```python
from build123d import *

# Parameters (mm, degrees)
SKETCH1_W                      = 16
SKETCH1_H                      = 40
BOSS_EXTRUDE1_DEPTH            = 30
F_3_8_0_3750_DOWEL_HOLE1_D     = 9.525
F_1_8_0_1250_DOWEL_HOLE1_D     = 3.175
SKETCH7_W                      = 10
SKETCH7_H                      = 40
CUT_EXTRUDE1_DEPTH             = 15
F_3_16_0_1875_DIAMETER_HOLE1_D = 4.7625
SKETCH10_W                     = 16
SKETCH10_H                     = 23.65
CUT_EXTRUDE2_DEPTH             = 15
FILLET1_R                      = 10


with BuildPart() as part:
    # Sketch1 → Boss-Extrude1 (new body)
    with BuildSketch(Plane.XY):
        with Locations((0, -10)):
            Rectangle(SKETCH1_W, SKETCH1_H)
    extrude(amount=BOSS_EXTRUDE1_DEPTH)

    # 3/8 (0.3750) Dowel Hole1 (through all)
    with Locations(Plane.XY.offset(30)):
        with Locations((0, 0)):
            Hole(F_3_8_0_3750_DOWEL_HOLE1_D / 2)

    # 1/8 (0.1250) Dowel Hole1 (through all)
    with Locations(Plane.ZY.offset(8)):
        with Locations((7.5, 0)):
            Hole(F_1_8_0_1250_DOWEL_HOLE1_D / 2)

    # Sketch7 → Cut-Extrude1 (cut)
    with BuildSketch(Plane.XY.offset(30)):
        with Locations((0, -10)):
            Rectangle(SKETCH7_W, SKETCH7_H)
    extrude(amount=-CUT_EXTRUDE1_DEPTH, mode=Mode.SUBTRACT)

    # 3/16 (0.1875) Diameter Hole1 (through all)
    with Locations(Plane.ZY.offset(8)):
        with Locations((22, -2), (22, -23.7)):
            Hole(F_3_16_0_1875_DIAMETER_HOLE1_D / 2)

    # Sketch10 → Cut-Extrude2 (cut)
    with BuildSketch(Plane(origin=(0, 0, 0), x_dir=(-1, 0, 0), z_dir=(0, 0, -1))):
        with Locations((0, -18.175)):
            Rectangle(SKETCH10_W, SKETCH10_H)
    extrude(amount=-CUT_EXTRUDE2_DEPTH, mode=Mode.SUBTRACT)

    # Fillet1
    fillet1_edges = [part.edges().sort_by_distance(p)[0] for p in [
        (6.5, 10, 30),
        (6.5, -30, 30),
        (-6.5, 10, 30),
        (-6.5, -30, 30),
    ]]
    fillet(fillet1_edges, radius=FILLET1_R)


solid = part.part
```
Build history of the part. All positions in model axes, mm. A direction names the side the tool comes from. Coordinates: 2 decimals unless noted, no trailing zeros. Order: outer loops, then holes, each group sorted by start corner. A loop starts at its lowest first (then second) coordinate and runs counter-clockwise, first axis right, second up.
Item 1: Drill centre lines: L1, parallel to Y at x = -0.25, z = 5; L2, parallel to Y at x = 6.1, z = 22; L3, parallel to X at y = -6.5, z = 29. Where is each one in solid material? Low to high.
Filled in:
L1: y = -6.35 to -4.76, 4.76 to 10
L2: y = -29.8 to -26.08, -21.32 to -4.38, 0.38 to 9.8
L3: x = -8 to -5, 5 to 8
Item 2: Mould opens along X. For faces 3 (the cylindrical face through (6.52, -1.28, 19.73)), 4 (the flat face through (5, -10, 23)), 5 (the flat face through (8, -6, 18)), 6 (the cylindrical face through (-4.4, -1.82, 7.39)) say: released by +X, released by -X, zero draft, split by the parting line, or undercut.
Filled in:
face 3: zero draft
face 4: undercut
face 5: released by +X
face 6: undercut
Item 3: Saw through at A-A on z = 15.5. List the corners of the cut face in (x, y), then the cut area to 3 significant figures.
Filled in:
outline: (-8, -30) - (-5, -30) - (-5, 10) - (-8, 10) - close; (5, -30) - (8, -30) - (8, 10) - (5, 10) - close
area: 240 mm2
Item 4: Tool access for faces 1 (the cylindrical face through (6.52, -25.81, 20.9)), 2 (the flat face through (0, -6.35, 7)): list every direction of +Z, -Z, +X, -X, +Y, -Y with a clear straight run to the whole face (end or side of a thin tool).
Filled in:
face 1: +X, -X
face 2: -Z, +X, -X, -Y
Item 5: Saw through at C-C on x = 0. List the corners of the cut face in (y, z), then the cut area to 3 significant figures.
Filled in:
outline: (-6.35, 0) - (-4.76, 0) - (-4.76, 15) - (-6.35, 15) - close; (4.76, 0) - (10, 0) - (10, 15) - (4.76, 15) - close
area: 102 mm2
Item 6: Saw through at B-B on y = 1. List the corners of the cut face in (x, z).
Filled in:
outline: (-8, 0) - (-4.66, 0) - (-4.66, 6.27) - (-8, 6.27) - close; (-8, 8.73) - (-4.66, 8.73) - (-4.66, 15) - (-5, 15) - (-5, 29.95) - (-8, 29.95) - close; (4.66, 0) - (8, 0) - (8, 6.27) - (4.66, 6.27) - close; (4.66, 8.73) - (8, 8.73) - (8, 29.95) - (5, 29.95) - (5, 15) - (4.66, 15) - close
Item 7: Saw through at D-D on x = -5.5. State how many separate pieces and enclosed holes the cut face has, then the cut area to 3 significant figures.
Filled in:
separate pieces: 1
enclosed holes: 3
area: 759 mm2
Item 8: Drop flat-ended pins along their axis: pin 1 Ø3 at (y, z) = (-2, 22) entering from +X; pin 2 Ø2.5 at (x, y) = (-7, -23) entering from -Z. Give the stop position or say it passes through.
Filled in:
pin 1: passes through
pin 2: stops at z = 15
